Here's how the part is built. I have some questions about the finished solid (model axes, mm). Round coordinates to 2 decimals unless told otherwise and drop trailing zeros. Order: outer loops, then holes, each group sorted by start corner. A loop starts at its lowest first (then second) coordinate and runs counter-clockwise, first axis right, second up.
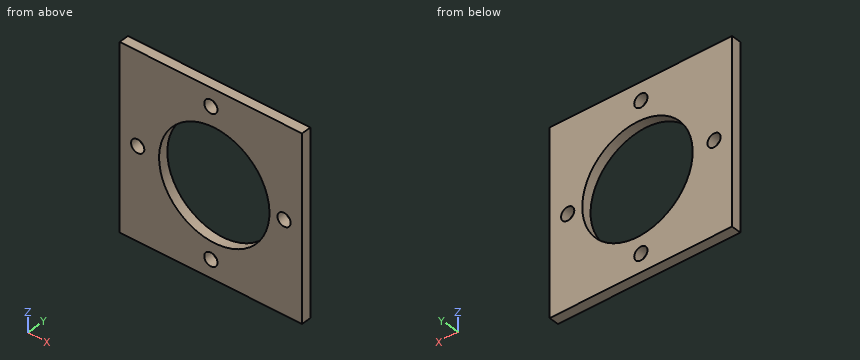
```python
from build123d import *

# Parameters (mm, degrees)
SKETCH1_W           = 82.6
SKETCH1_H           = 82.6
BOSS_EXTRUDE1_DEPTH = 4.47
SKETCH5_R           = 25
CUT_EXTRUDE2_DEPTH  = 117.899533361
SKETCH7_R           = 3
CUT_EXTRUDE3_DEPTH  = 117.899533361


with BuildPart() as part:
    # Sketch1 → Boss-Extrude1 (new body)
    with BuildSketch(Plane(origin=(0, 0, 0), x_dir=(1, 0, 0), z_dir=(0, 1, 0))):
        with Locations((41.3, 41.3)):
            Rectangle(SKETCH1_W, SKETCH1_H)
    extrude(amount=BOSS_EXTRUDE1_DEPTH)

    # Sketch5 → Cut-Extrude2 (cut, through all)
    with BuildSketch(Plane(origin=(0, 4.47, 0), x_dir=(1, 0, 0), z_dir=(0, 1, 0))):
        with Locations(Location((42.841926389, 41.575343998, 0), (0, 0, 270))):
            Circle(SKETCH5_R)
    extrude(amount=-CUT_EXTRUDE2_DEPTH, mode=Mode.SUBTRACT)

    # Sketch7 → Cut-Extrude3 (cut, through all)
    with BuildSketch(Plane(origin=(0, 4.47, 0), x_dir=(1, 0, 0), z_dir=(0, 1, 0))):
        with Locations(Location((8.15, 41.3, 0), (0, 0, 270))):
            Circle(SKETCH7_R)
        with Locations(Location((41.3, 74.45, 0), (0, 0, 270))):
            Circle(SKETCH7_R)
        with Locations(Location((74.45, 41.3, 0), (0, 0, 270))):
            Circle(SKETCH7_R)
        with Locations(Location((41.3, 8.15, 0), (0, 0, 270))):
            Circle(SKETCH7_R)
    extrude(amount=-CUT_EXTRUDE3_DEPTH, mode=Mode.SUBTRACT)


solid = part.part
```
1. If we section it at B-B, the plane z = -8.15: Write out the boundary of the cut face in (x, y), and give its area (3 significant figures).
Evaluation:
outline: (0, 0) - (38.3, 0) - (38.3, 4.47) - (0, 4.47) - close; (44.3, 0) - (82.6, 0) - (82.6, 4.47) - (44.3, 4.47) - close
area: 342 mm2
2. If we section it at D-D, the plane z = -42: Write out the boundary of the cut face in (x, y), and give its area (3 significant figures).
Evaluation:
outline: (0, 0) - (5.23, 0) - (5.23, 4.47) - (0, 4.47) - close; (11.07, 0) - (17.85, 0) - (17.85, 4.47) - (11.07, 4.47) - close; (67.84, 0) - (71.53, 0) - (71.53, 4.47) - (67.84, 4.47) - close; (77.37, 0) - (82.6, 0) - (82.6, 4.47) - (77.37, 4.47) - close
area: 93.6 mm2
3. I'm going to push a flat-ended pin straight in: P1, Ø8, axis at x = 44.5, z = -24, coming from the +Y side. Where does the tip first touch, or does it pass through?
Evaluation:
P1: passes through
4. If we section it at C-C, the plane y = 0.8: Write out the boundary of the cut face in (x, z), and give its area (3 significant figures).
Evaluation:
outline: (0, -82.6) - (82.6, -82.6) - (82.6, 0) - (0, 0) - close; hole circle Ø6 at (8.15, -41.3); hole circle Ø50 at (42.84, -41.58); hole circle Ø6 at (41.3, -74.45); hole circle Ø6 at (41.3, -8.15); hole circle Ø6 at (74.45, -41.3)
area: 4,750 mm2
5. If we section it at A-A, the plane x = 8.15: Write out the boundary of the cut face in (y, z).
Evaluation:
outline: (0, -82.6) - (4.47, -82.6) - (4.47, -44.3) - (0, -44.3) - close; (0, -38.3) - (4.47, -38.3) - (4.47, 0) - (0, 0) - close
6. I need wall thicknesses on probe 1 along X at (y, z) = (2.75, -8.15); probe 2 along Z at (x, y) = (43, 4.2); probe 3 along X at (y, z) = (3.75, -59). Which ranges of each line are inside material? Lowest first, please.
Evaluation:
probe 1: x = 0 to 38.3, 44.3 to 82.6
probe 2: z = -82.6 to -76.92, -71.98 to -66.57, -16.58 to -10.62, -5.68 to 0
probe 3: x = 0 to 24.91, 60.77 to 82.6
